```python
from build123d import *

# Parameters (mm, degrees)
BOSS_EXTRUDE3_DEPTH = 200
SKETCH5_W           = 135
SKETCH5_H           = 7.5
CUT_EXTRUDE1_DEPTH  = 5
SKETCH6_W           = 20
SKETCH6_H           = 45
BOSS_EXTRUDE4_DEPTH = 25
SKETCH7_W           = 5
SKETCH7_H           = 7.5
CUT_EXTRUDE2_DEPTH  = 175


with BuildPart() as part:
    # Sketch4 → Boss-Extrude3 (new body)
    with BuildSketch(Plane.XY):
        Polygon((5, -3.75), (0, -3.75), (0, -22.5), (-15, -22.5), (-15, 22.5), (0, 22.5), (0, 3.75), (5, 3.75), align=None)
    extrude(amount=BOSS_EXTRUDE3_DEPTH)

    # Sketch5 → Cut-Extrude1 (cut)
    with BuildSketch(Plane(origin=(5, 0, 0), x_dir=(0, 0, -1), z_dir=(1, 0, 0))):
        with Locations((-132.5, 0)):
            Rectangle(SKETCH5_W, SKETCH5_H)
    extrude(amount=-CUT_EXTRUDE1_DEPTH, mode=Mode.SUBTRACT)

    # Sketch6 → Boss-Extrude4 (add)
    with BuildSketch(Plane.XY.offset(200)):
        with Locations((-25, 0)):
            Rectangle(SKETCH6_W, SKETCH6_H)
    extrude(amount=-BOSS_EXTRUDE4_DEPTH)

    # Sketch7 → Cut-Extrude2 (cut)
    with BuildSketch(Plane(origin=(0, 0, 0), x_dir=(-1, 0, 0), z_dir=(0, 0, -1))):
        with Locations((12.5, 0)):
            Rectangle(SKETCH7_W, SKETCH7_H)
    extrude(amount=-CUT_EXTRUDE2_DEPTH, mode=Mode.SUBTRACT)


solid = part.part
```
Geometry: final body of the model. Coordinates: model frame, mm. A direction names the side the tool comes from. Round coordinates to 2 decimals unless told otherwise and drop trailing zeros. Order: outer loops, then holes, each group sorted by start corner. A loop starts at its lowest first (then second) coordinate and runs counter-clockwise, first axis right, second up. Notation, with made-up numbers: M 52,11 L 90,11 A4 ccw 90,17 Z; hole C -1,-3.75 d6. An arc over 180 degrees is marked long. One line per item, written item: value.
(1) Cut plane B-B (z = 151.5). Return the cut outline in (x, y), and give its area (4 significant figures).
Result sheet:
outline: M -15,-22.5 L 0,-22.5 L 0,22.5 L -15,22.5 L -15,3.75 L -10,3.75 L -10,-3.75 L -15,-3.75 Z
area: 637.5 mm2
(2) Cut plane C-C (x = -26). Return the cut outline in (y, z), and give its area (4 significant figures).
Result sheet:
outline: M -22.5,175 L 22.5,175 L 22.5,200 L -22.5,200 Z
area: 1,125 mm2
(3) Line query: probe 1 along Y at (x, z) = (-10.5, 46); probe 2 along Z at (x, y) = (-22.5, 4.5); probe 3 along X at (y, z) = (7.5, 159.5). Output: solid intervals per line, ascending. Write a range as [from, to].
Result sheet:
probe 1: [-22.5, -3.75], [3.75, 22.5]
probe 2: [175, 200]
probe 3: [-15, 0]
(4) Pin query (flat end, axial travel): P1, Ø1.5, axis at y = 7, z = 155.5, coming from the +X side; P2, Ø20.5, axis at y = -12.5, z = 63, coming from the -X side; P3, Ø5, axis at x = -19.5, y = 11.5, coming from the -Z side. Return the tip coordinate at first contact, or that it passes through.
Result sheet:
P1: x = 0
P2: x = -15
P3: z = 175
(5) Cut plane D-D (z = 52). Return the cut outline in (x, y).
Result sheet:
outline: M -15,-22.5 L 0,-22.5 L 0,-3.75 L 5,-3.75 L 5,3.75 L 0,3.75 L 0,22.5 L -15,22.5 L -15,3.75 L -10,3.75 L -10,-3.75 L -15,-3.75 Z
(6) Pull-direction query (Y, two-part tool) for faces 5 (the flat face through (3, -3.75, 32)), 6 (the flat face through (-12, 3.75, 86)), 7 (the flat face through (-18, 0, 200)), 8 (the flat face through (-10, 0, 86)); classes: pulls with the +Y half, pulls with the -Y half, needs draft (parallel to the pull), parting line crosses it, or undercut.
Result sheet:
face 5: pulls with the -Y half
face 6: undercut
face 7: needs draft
face 8: undercut
(7) Reachability of faces 1 (the flat face through (3, 0, 65)), 2 (the flat face through (2, 3.75, 32)), 3 (the flat face through (-15, -13, 86)), 4 (the flat face through (-12, -3.75, 86)) from +Z, -Z, +X, -X, +Y, -Y: full face, straight path, thin tool, end or side. Return the list, or none.
Result sheet:
face 1: +Z, +X, +Y, -Y
face 2: +Z, -Z, +X, +Y
face 3: -Z, -X, +Y, -Y
face 4: -Z, -X
(8) Cut plane A-A (y = -0.5). Return the cut outline in (x, z).
Result sheet:
outline: M -35,175 L -10,175 L -10,0 L 5,0 L 5,65 L 0,65 L 0,200 L -35,200 Z
